Autodesk Inventor part; units mm, degrees
ref_plane "YZ Plane" through (0, 0, 0) normal (1, 0, 0) x (0, 1, 0)
ref_plane "XZ Plane" through (0, 0, 0) normal (0, 1, 0) x (-1, 0, 0)
ref_plane "XY Plane" through (0, 0, 0) normal (0, 0, 1) x (1, 0, 0)
sketch "Sketch1" plane through (0, 0, 0) normal (0, 1, 0) x (-1, 0, 0)
  circle A0 centre (0, 0) radius 50.8
  dimension "d0" = 101.6
extrude "Extrusion1" add sketch "Sketch1" along normal blind 406.4
sketch "Sketch2" plane through (0, 0, 0) normal (1, 0, 0) x (0, 1, 0)
  line L0 (0, -50.8) -> (0, 50.8)
  line L1 (12.7, 19.05) -> (50.8, 19.05)
  line L2 (50.8, 19.05) -> (50.8, -19.05)
  line L3 (50.8, -19.05) -> (12.7, -19.05)
  line L4 (12.7, -19.05) -> (12.7, 19.05)
  point P0 (0, 0)
  dimension "d5" = 38.1
  dimension "d6" = 38.1
extrude "Extrusion2" cut sketch "Sketch2" along normal blind 101.6
sketch "Sketch3" plane through (0, 406.4, 0) normal (0, 1, 0) x (1, 0, 0)
  circle A0 centre (0, 0) radius 19.05
  dimension "d9" = 38.1
extrude "Extrusion3" cut sketch "Sketch3" against normal blind 393.7
properties part number "Shaft Connecting Chassis"
Can you work these out from the model? Positions are in its coordinate system, mm. A direction names the side the tool comes from. Coordinates: 2 decimals unless noted, no trailing zeros. Order: outer loops, then holes, each group sorted by start corner. A loop starts at its lowest first (then second) coordinate and runs counter-clockwise, first axis right, second up. Notation, with made-up numbers: (-14, 8.5) - (9, 8.5) arc R29 cw to (9, 29.5) - close; hole circle Ø6 at (52, 73.5). An arc over 180 degrees is marked (long way). Answer as a JSON object with one key per item and string values. Group by question number.
Q1. On a 3-axis mill with a long thin cutter (end or side, diameter ignored), from which of +Z, -Z, +X, -X, +Y, -Y can I reach the whole of each face in a straight line? I mean faces 4 (the face through (23, 31, 19.05)), 5 (the face through (1, 0, 1)). Say none if no direction works.
Q2. Imagine slicing it at A-A (z = 0). Please give me the cut outline in (x, y), and give its area (3 significant figures).
Q3. Imagine slicing it at B-B (x = 28.5). Please give me the cut outline in (y, z).
Q4. I need wall thicknesses on line 1 (X direction, y = 248.5, z = 0); line 2 (Y direction, x = -10.5, z = -5). Which ranges of each line are inside material? Lowest first, please. Write a range as from..to.
Q5. We'd pull the mould along X, two halves only. Please class faces 1 (the face through (-22, 406.4, 1)), 2 (the face through (-19.03, 212.31, -0.84)), 3 (the face through (-48.454, 200.355, -15.259)): +X half, -X half, draft (parallel to the pull), parting line (faces both ways), or undercut.
Q6. Imagine slicing it at C-C (y = 182). Please give me the cut outline in (x, z), and give its area (3 significant figures).
Q7. Imagine slicing it at D-D (x = -6). Please give me the cut outline in (y, z).
Q8. Will these pins go through, and if not, where does the flat tip stop? P1, Ø2, axis at x = -25.5, y = 158, coming from the -Z side; P2, Ø5, axis at y = 220.5, z = 23, coming from the -X side; P3, Ø1.5, axis at x = 18, y = 204, coming from the +Z side.
Determined:
{
 "1": {"face 4": "+X", "face 5": "+Z, -Z, +X, -X, -Y"},
 "2": {"outline": "(-50.8, 0) - (50.8, 0) - (50.8, 12.7) - (-19.05, 12.7) - (-19.05, 406.4) - (-50.8, 406.4) - close; (19.05, 50.8) - (50.8, 50.8) - (50.8, 406.4) - (19.05, 406.4) - close", "area": "25,100 mm2"},
 "3": {"outline": "(0, -42.05) - (406.4, -42.05) - (406.4, 42.05) - (0, 42.05) - close; hole (12.7, -19.05) - (50.8, -19.05) - (50.8, 19.05) - (12.7, 19.05) - close"},
 "4": {"line 1": "x = -50.8..-19.05, 19.05..50.8", "line 2": "y = 0..12.7"},
 "5": {"face 1": "draft", "face 2": "undercut", "face 3": "parting line"},
 "6": {"outline": "circle Ø101.6 at (0, 0); hole circle Ø38.1 at (0, 0)", "area": "6,970 mm2"},
 "7": {"outline": "(0, -50.44) - (406.4, -50.44) - (406.4, -18.08) - (12.7, -18.08) - (12.7, 18.08) - (406.4, 18.08) - (406.4, 50.44) - (0, 50.44) - close"},
 "8": {"P1": "stops at z = -44.5", "P2": "stops at x = -46.48", "P3": "stops at z = 47.78"}
}
